from build123d import *

# Parameters (mm, degrees)
AUFSATZ_LINEAR_AUSTRAGEN1_DEPTH = 7
SKIZZE4_R                       = 6
AUFSATZ_LINEAR_AUSTRAGEN3_DEPTH = 7
SKIZZE5_R                       = 3.5
SCHNITT_LINEAR_AUSTRAGEN1_DEPTH = 38.075373678


with BuildPart() as part:
    # Skizze1 → Aufsatz-Linear austragen1 (new body)
    with BuildSketch(Plane(origin=(0, 0, 0), x_dir=(1, 0, 0), z_dir=(0, 1, 0))):
        Polygon((8.082903769, 0), (4.041451884, 7), (-4.041451884, 7), (-8.082903769, 0), (-4.041451884, -7), (4.041451884, -7), align=None)
    extrude(amount=AUFSATZ_LINEAR_AUSTRAGEN1_DEPTH)

    # Skizze3 → Rotation1 (revolve)
    with BuildSketch(Plane.XY, mode=Mode.PRIVATE) as rotation1_sk:
        Polygon((0, 7), (-6, 7), (-6, 16), (-5, 17), (-5, 18.5), (-6, 20), (-6, 21.5), (-5, 22.5), (-5, 28.5), (0, 28.5), align=None)
    revolve(rotation1_sk.sketch.rotate(Axis((0, 0, 0), (0, 1, 0)), 270), axis=Axis((0, 0, 0), (0, 1, 0)))

    # Skizze4 → Aufsatz-Linear austragen3 (add)
    with BuildSketch(Plane.XZ):
        with Locations(Location((0, 0, 0), (0, 0, 270))):
            Circle(SKIZZE4_R)
    extrude(amount=AUFSATZ_LINEAR_AUSTRAGEN3_DEPTH)

    # Skizze5 → Schnitt-Linear austragen1 (cut, through all)
    with BuildSketch(Plane(origin=(0, 28.5, 0), x_dir=(1, 0, 0), z_dir=(0, 1, 0))):
        with Locations(Location((0, 0, 0), (0, 0, 270))):
            Circle(SKIZZE5_R)
    extrude(amount=-SCHNITT_LINEAR_AUSTRAGEN1_DEPTH, mode=Mode.SUBTRACT)


solid = part.part
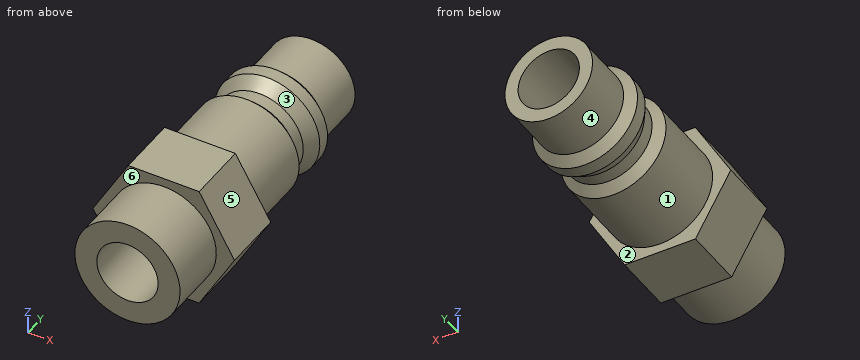
Part model, mm, in its own coordinate system. Face numbers are marked on the shaded views. A direction names the side the tool comes from. Coordinates: 2 decimals unless noted, no trailing zeros. Loops run counter-clockwise (first coordinate to the right, second up) from the corner with the lowest first, then second, coordinate; pieces in that order, holes last. Notation, with made-up numbers: (-34, 36) -> (23, 36) arc R23 cw to (23, 74) -> close; hole circle Ø1 at (66.5, 40). An arc over 180 degrees is marked (long way). Use a Markdown table: item, result. Add a question column.
Item 1: Which spindle directions (+Z, -Z, +X, -X, +Y, -Y) get a long thin tool onto all of the face, cutting with end or side? Do the marked faces 4, 5 and 6. Say none if no direction does.
Item 2: Flat gauge pins, fed straight in: P1, Ø1, axis at x = 4, y = 24, coming from the -Z side; P2, Ø1, axis at x = -3, y = 13.5, coming from the -Z side; P3, Ø3, axis at x = -3.5, y = 18, coming from the +Z side. Where does each tip first touch, or does it go through?
Item 3: Probe probe 1 along X at (y, z) = (11.5, 0); probe 2 along Y at (x, z) = (4.5, 5.5); probe 3 along Z at (x, y) = (1, 15.5). List the from-to ranges inside material, lowest first.
Item 4: Pull direction Y, two halves, no side cores. Call the marked faces 1, 2 and 3: +Y half, -Y half, draft (parallel to the pull), parting line (faces both ways), or undercut.
Item 5: Band-saw the part on C-C on y = -1.5. Write the cut outline in (x, z), plus the area to 3 significant figures.
Item 6: Band-saw the part on D-D on y = 25. Write the cut outline in (x, z).
Item 7: Band-saw the part on A-A on x = 0. Write the cut outline in (y, z).
Item 8: Band-saw the part on B-B on y = 4. Write the cut outline in (x, z).
Geometry says:
| question | item | result |
|---|---|---|
| 1 | face 4 | +Y |
| 1 | face 5 | +Z, +X, +Y, -Y |
| 1 | face 6 | -Y |
| 2 | P1 | z = -3.57 |
| 2 | P2 | z = -5.45 |
| 2 | P3 | z = 4.81 |
| 3 | probe 1 | -6 to -3.5, 3.5 to 6 |
| 3 | probe 2 | 0 to 7 |
| 3 | probe 3 | -5.92 to -3.35, 3.35 to 5.92 |
| 4 | face 1 | draft |
| 4 | face 2 | +Y half |
| 4 | face 3 | undercut |
| 5 | outline | circle Ø12 at (0, 0); hole circle Ø7 at (0, 0) |
| 5 | area | 74.6 mm² |
| 6 | outline | circle Ø10 at (0, 0); hole circle Ø7 at (0, 0) |
| 7 | outline | (-7, -6) -> (0, -6) -> (0, -7) -> (7, -7) -> (7, -6) -> (16, -6) -> (17, -5) -> (18.5, -5) -> (20, -6) -> (21.5, -6) -> (22.5, -5) -> (28.5, -5) -> (28.5, -3.5) -> (-7, -3.5) -> close; (-7, 3.5) -> (28.5, 3.5) -> (28.5, 5) -> (22.5, 5) -> (21.5, 6) -> (20, 6) -> (18.5, 5) -> (17, 5) -> (16, 6) -> (7, 6) -> (7, 7) -> (0, 7) -> (0, 6) -> (-7, 6) -> close |
| 8 | outline | (-8.08, 0) -> (-4.04, -7) -> (4.04, -7) -> (8.08, 0) -> (4.04, 7) -> (-4.04, 7) -> close; hole circle Ø7 at (0, 0) |
